Input: part model. Units: mm. Frame: model coordinates. A direction names the side the tool comes from. Round coordinates to 2 decimals unless told otherwise and drop trailing zeros. Loops run counter-clockwise (first coordinate to the right, second up) from the corner with the lowest first, then second, coordinate; pieces in that order, holes last. Notation, with made-up numbers: (34.5, 53.5) -> (45.5, 53.5) arc R21 cw to (45.5, 80.5) -> close; hole circle Ø3 at (-31.75, 2). An arc over 180 degrees is marked (long way). One line per question, with ' | ' between items. Start each with the question number.
Q1. Cut plane A-A on y = 0. Return loops of the section in (x, z).
Q2. Access query for faces 1 (the face through (4.95, 0, 13)), 2 (the face through (-4, 4, 15)). Directions: +Z, -Z, +X, -X, +Y, -Y. A direction counts if a zero-diameter tool reaches every point of the face in a straight line with its end or side. Return the directions, or none.
Q3. Cut plane C-C on z = 3.75. Return loops of the section in (x, y).
Q4. Cut plane B-B on z = 11.25. Return loops of the section in (x, y), and give its area (3 significant figures).
Q5. Contact query for flat-ended pins moving along their axis: P1, Ø1.5, axis at x = 9, z = 9.5, coming from the +Y side; P2, Ø1.5, axis at x = 3, z = 13, coming from the -Y side. Output: stop coordinate, or through.
Q6. Material intervals for L1, parallel to Y at x = 0, z = 3.5; L2, parallel to Z at x = -15.5, y = -2; L3, parallel to X at y = -1, z = 2, sorted ascending.
Q7. Mould query, pull axis X, two halves, no side actions, for faces 3 (the face through (-2.51, -4.267, 12.535)), 4 (the face through (-13.887, -10.648, 6.409)), 5 (the face through (-3.4, -1.2, 10)), 6 (the face through (0, -4, 0)). Classes: pulls with the +X half, pulls with the -X half, needs draft (parallel to the pull), parting line crosses it, or undercut.
from build123d import *

# Parameters (mm, degrees)
F0_R     = 17.5
F1_DEPTH = 15
F3_DEPTH = 5
F4_R     = 2
F5_R     = 3.4
F6_DEPTH = 10.001


with BuildPart() as f1:
    # F0 (on Top) → F1 (new body)
    with BuildSketch(Plane.XY):
        Circle(F0_R)
    extrude(amount=F1_DEPTH)

    # F2 (on face) → F3 (cut)
    with BuildSketch(Plane.XY.offset(15)):
        Polygon((0, -5.715768), (4.95, -2.857884), (4.95, 2.857884), (0, 5.715768), (-4.95, 2.857884), (-4.95, -2.857884), align=None)
    extrude(amount=-F3_DEPTH, mode=Mode.SUBTRACT)

    # F4
    f4_edges = [f1.edges().sort_by_distance(p)[0] for p in [
        (-17.5, 0, 15),
    ]]
    fillet(f4_edges, radius=F4_R)

    # F5 (on face) → F6 (cut, through all)
    with BuildSketch(Plane.XY.offset(10)):
        Circle(F5_R)
    extrude(amount=-F6_DEPTH, mode=Mode.SUBTRACT)


solid = f1.part
Results:
1) outline: (-17.5, 0) -> (-3.4, 0) -> (-3.4, 10) -> (-4.95, 10) -> (-4.95, 15) -> (-15.5, 15) arc R2 ccw to (-17.5, 13) -> close; (3.4, 0) -> (17.5, 0) -> (17.5, 13) arc R2 ccw to (15.5, 15) -> (4.95, 15) -> (4.95, 10) -> (3.4, 10) -> close
2) face 1: +Z | face 2: +Z, +X, -X, +Y, -Y
3) outline: circle Ø35 at (0, 0); hole circle Ø6.8 at (0, 0)
4) outline: circle Ø35 at (0, 0); hole (-4.95, -2.86) -> (0, -5.72) -> (4.95, -2.86) -> (4.95, 2.86) -> (0, 5.72) -> (-4.95, 2.86) -> close | area: 877 mm^2
5) P1: y = 15.43 | P2: y = -17.35
6) L1: -17.5 to -3.4, 3.4 to 17.5 | L2: 0 to 15 | L3: -17.47 to -3.25, 3.25 to 17.47
7) face 3: undercut | face 4: parting line crosses it | face 5: undercut | face 6: needs draft
